Could you check a few things on this drawing? It's one solid part, dimensions in mm from its lowest x, y, z. A direction names the side the tool comes from. Give positions to 0.01 mm unless a question says otherwise; leave off trailing zeros. Loops run counter-clockwise (first coordinate to the right, second up) from the corner with the lowest first, then second, coordinate; pieces in that order, holes last. Notation, with made-up numbers: M 46.5,31.5 L 57.5,31.5 A14 ccw 57.5,39.5 Z; hole C 28.5,55 d9. An arc over 180 degrees is marked long. Answer in a Markdown table with one row per item. Add a question column.
1. If we section it at B-B on y = 11.5: List the corners of the cut face in (x, z) for me (3 decimals).
2. If we section it at A-A on z = 13.5: List the corners of the cut face in (x, y) for me.
3. I'm going to push flat-ended pins straight in: pin 1 Ø1.5 at (y, z) = (42, 4.5) entering from -X; pin 2 Ø3 at (y, z) = (56, 5.5) entering from +X; pin 3 Ø14.5 at (y, z) = (22, 21.5) entering from +X. Where does each tip first touch, or does it pass through?
4. Thinking about a two-plate mould opening in X: for the marked faces 1, 2, 3 and 4, which applies, released by +X, released by -X, zero draft, split by the parting line, or undercut?
5. If we section it at C-C on x = 63.5: List the corners of the cut face in (y, z) for me.
6. I need wall thicknesses on line 1 along Y through (x, z) = (63.5, 18); line 2 along Y through (x, z) = (63, 9); line 3 along X through (y, z) = (16, 11). Which ranges of each line are inside material? Lowest first, please. Write a range as from..to.
7. If we section it at D-D on y = 36.5: List the corners of the cut face in (x, z) for me.
8. Which directions (+Z, -Z, +X, -X, +Y, -Y) give clear straight access to the entire face, cutting with the end or side of a thin tool? Please do the marked faces 5, 6 and 7.
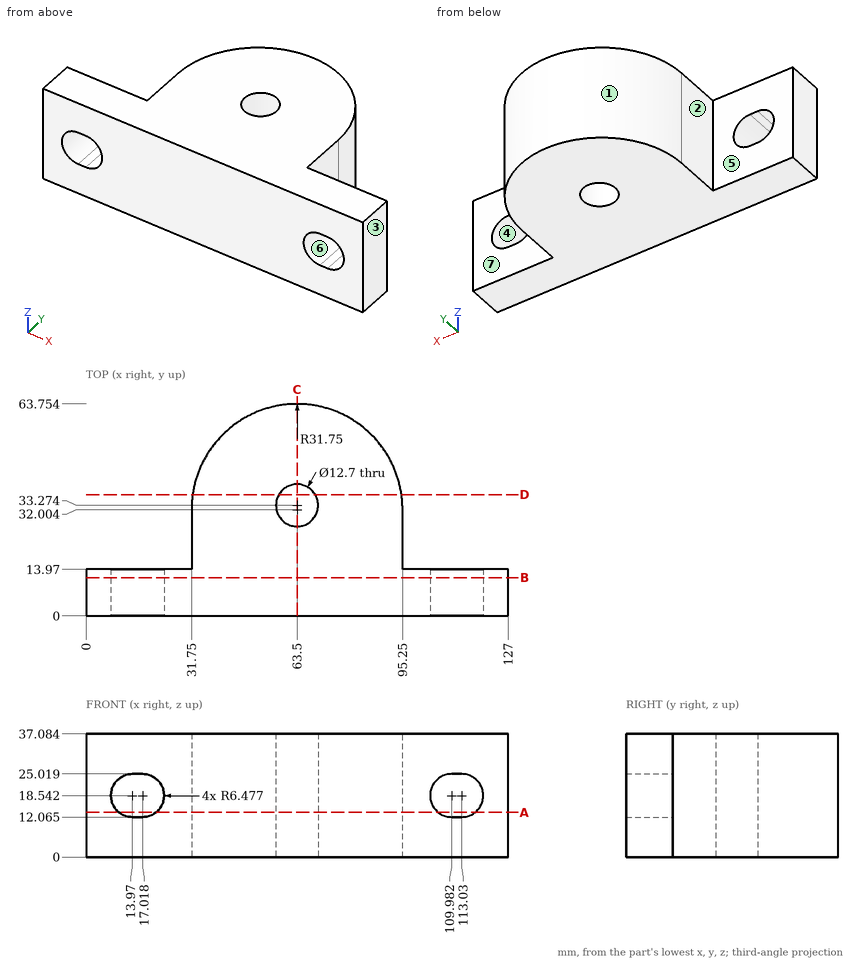
Results:
| question | item | result |
|---|---|---|
| 1 | outline | M 0,0 L 127,0 L 127,37.084 L 0,37.084 Z; hole M 13.97,12.065 L 17.018,12.065 A6.477 ccw 17.018,25.019 L 13.97,25.019 A6.477 ccw Z; hole M 109.982,12.065 L 113.03,12.065 A6.477 ccw 113.03,25.019 L 109.982,25.019 A6.477 ccw Z |
| 2 | outline | M 0,0 L 9.9,0 L 9.9,13.97 L 0,13.97 Z; M 21.08,0 L 105.92,0 L 105.92,13.97 L 95.25,13.97 L 95.25,32 A31.75 ccw 31.75,32 L 31.75,13.97 L 21.08,13.97 Z; M 117.1,0 L 127,0 L 127,13.97 L 117.1,13.97 Z; hole C 63.5,33.27 d12.7 |
| 3 | pin 1 | x = 33.13 |
| 3 | pin 2 | x = 85.91 |
| 3 | pin 3 | x = 95.25 |
| 4 | face 1 | split by the parting line |
| 4 | face 2 | released by -X |
| 4 | face 3 | released by +X |
| 4 | face 4 | undercut |
| 5 | outline | M 0,0 L 26.92,0 L 26.92,37.08 L 0,37.08 Z; M 39.62,0 L 63.75,0 L 63.75,37.08 L 39.62,37.08 Z |
| 6 | line 1 | 0..26.92, 39.62..63.75 |
| 6 | line 2 | 0..26.94, 39.6..63.75 |
| 6 | line 3 | 31.75..95.25 |
| 7 | outline | M 32.07,0 L 58.03,0 L 58.03,37.08 L 32.07,37.08 Z; M 68.97,0 L 94.93,0 L 94.93,37.08 L 68.97,37.08 Z |
| 8 | face 5 | +Z, -Z, -X, +Y |
| 8 | face 6 | +Y, -Y |
| 8 | face 7 | +Z, -Z, +X, +Y |
